Print and shaded views of the part. All mm, measured from the part's lowest x, y and z. A direction names the side the tool comes from. Coordinates: 2 decimals unless noted, no trailing zeros. Loops run counter-clockwise (first coordinate to the right, second up) from the corner with the lowest first, then second, coordinate; pieces in that order, holes last. Notation, with made-up numbers: M -1,64 L 54,64 A23 cw 54,72 Z; hole C 43.5,76 d7. An arc over 180 degrees is marked long. Answer as a JSON object with one key per item and string values. Group by question number.
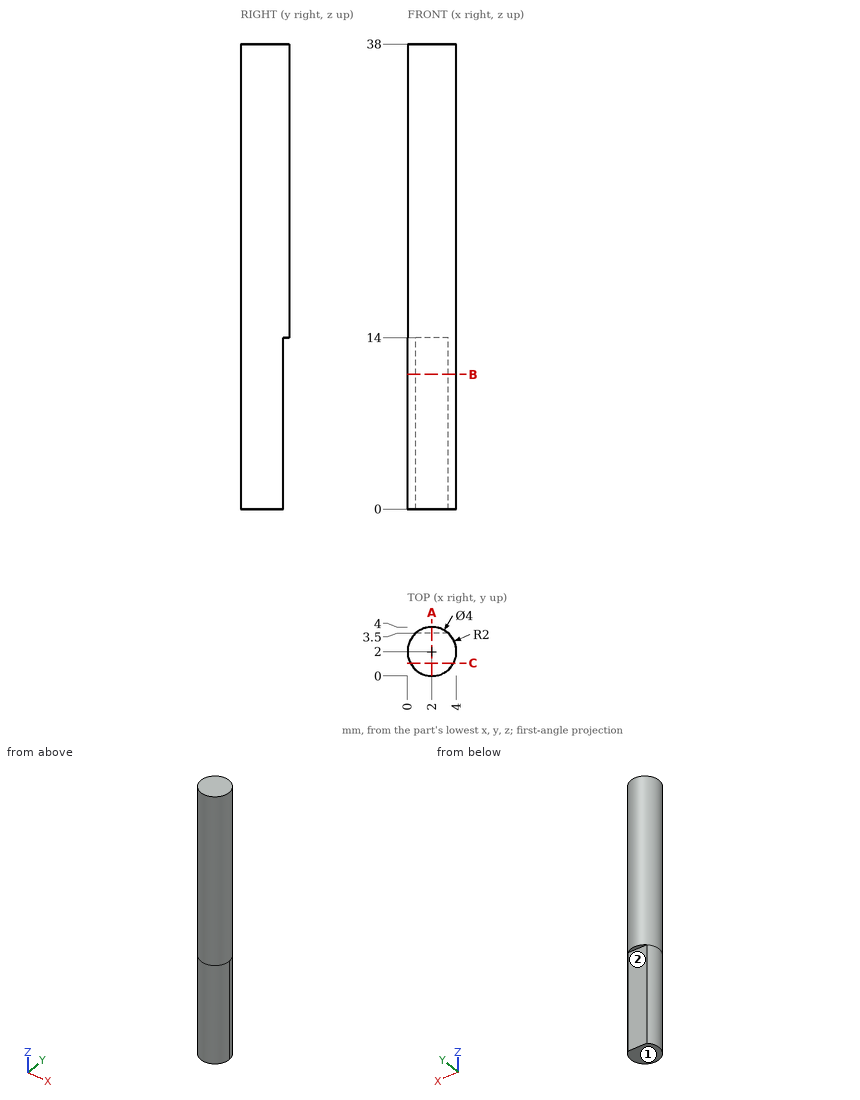
Item 1: Slice it at A-A, the plane x = 2. Write the cut outline in (y, z), then the cut area to 3 significant figures.
Item 2: Pin check, flat tips, straight feed: pin 1 (1.5 mm diameter, centred on x = 3, z = 20, fed in from -Y); pin 2 (1.3 mm diameter, centred on x = 1.5, z = 7, fed in from +Y); pin 3 (1 mm diameter, centred on y = 3, z = 23.5, fed in from -X). Stop position of each tip, or through.
Item 3: Slice it at C-C, the plane y = 1.05. Write the cut outline in (x, z), then the cut area to 3 significant figures.
Item 4: Tool access for the marked faces 1 and 2: list every direction of +Z, -Z, +X, -X, +Y, -Y with a clear straight run to the whole face (end or side of a thin tool).
Item 5: Drill centre lines: L1, parallel to X at y = 1.9, z = 7.5; L2, parallel to Y at x = 2.15, z = 26.5; L3, parallel to X at y = 0.6, z = 4. Where is each one in solid material? Low to high. Write a range as from..to.
Item 6: Slice it at B-B, the plane z = 11. Write the cut outline in (x, y), then the cut area to 3 significant figures.
Computed:
{
 "1": {"outline": "M 0,0 L 3.5,0 L 3.5,14 L 4,14 L 4,38 L 0,38 Z", "area": "145 mm2"},
 "2": {"pin 1": "y = 0.02", "pin 2": "y = 3.5", "pin 3": "x = 0.06"},
 "3": {"outline": "M 0.24,0 L 3.76,0 L 3.76,38 L 0.24,38 Z", "area": "134 mm2"},
 "4": {"face 1": "-Z, +X, -X, +Y, -Y", "face 2": "-Z, +X, -X, +Y"},
 "5": {"L1": "0..4", "L2": "0.01..3.99", "L3": "0.57..3.43"},
 "6": {"outline": "M 0.68,3.5 A2 ccw long 3.32,3.5 Z", "area": "11.7 mm2"}
}
